Check sheet for the modelled part. Datum: model origin and axes. Units: mm. A direction names the side the tool comes from. Round coordinates to 2 decimals unless told otherwise and drop trailing zeros. Order: outer loops, then holes, each group sorted by start corner. A loop starts at its lowest first (then second) coordinate and runs counter-clockwise, first axis right, second up.
Autodesk Fusion 360 part; units mm, degrees
sketch "Sketch1" plane through (0, 0, 0) normal (0, 0, 1) x (1, 0, 0)
  line L0 (0, 0) -> (280, 0)
  line L1 (280, 0) -> (280, -8)
  line L2 (280, -8) -> (0, -8)
  line L3 (0, -8) -> (0, 0)
  dimension "d1" = 280
  dimension "d2" = 8
extrude "Extrude1" add sketch "Sketch1" along normal blind 8
sketch "Sketch2" plane through (0, 0, 0) normal (0, 0, 1) x (1, 0, 0)
  circle A0 centre (280, -4) radius 12.5
  circle A1 centre (280, -4) radius 11.3
  dimension "d5" = 25
  dimension "d6" = 22.6
extrude "Extrude2" add sketch "Sketch2" along normal blind 8
extrude "Extrude3" cut sketch "Sketch2" along normal blind 8 contours A1
extrude "Extrude4" add sketch "Sketch2" along normal blind 1.2 contours A1
fillet "Fillet1" radius 5 1 edges at (269.4647, 0.0863, 1.2)
sketch "Sketch4" plane through (0, 0, 0) normal (0, 1, 0) x (-1, 0, 0)
  line L0 (-268.1573, 8) -> (-268.1573, 0)
  line L1 (-268.1573, 0) -> (0, 0)
  line L2 (0, 0) -> (0, 8)
  line L3 (0, 8) -> (-268.1573, 8)
  circle A0 centre (-5.4, 4.0245) radius 3.45
  circle A1 centre (-21.4, 3.9983) radius 2.05
  line L4 (-21.5827, 6.0402) -> (-5.7075, 7.4608)
  line L5 (-5.6963, 0.5873) -> (-21.576, 1.9559)
  dimension "d20" = 6.9
  dimension "d21" = 5.4
  dimension "d22" = 4.1
  dimension "d23" = 16
extrude "Extrude5" cut sketch "Sketch4" against normal blind 6 contours A0 | A0 A1 L4 L5 | A1
extrude "Extrude6" cut sketch "Sketch4" against normal blind 8 contours A0
fillet "Fillet2" radius 5 1 edges at (292.5, -4, 0)
fillet "Fillet3" radius 2 1 edges at (0, -4, 8)
fillet "Fillet4" radius 2 1 edges at (0, -4, 0)
equation "d6 = 25 mm - ( 1.2 * 2 ) * 1 mm"
equation "d21 = 3.4 mm + 2 mm"
1) Set-up check for faces 1 (the face through (271.12, 2.99, 7.09)), 2 (the face through (13.76, -2.96, 6.74)), 3 (the face through (136, -3, 8)): record each of +Z, -Z, +X, -X, +Y, -Y from which the full face is reachable in a straight line by a thin tool's end or side.
2) Scan lines: line 1 (Y direction, x = 280, z = 7.5); line 2 (Z direction, x = 5.4, y = -2.5); line 3 (Y direction, x = 104, z = 1.75). Record each from-to range of solid material in increasing order.
3) Draft check along X on faces 4 (the face through (292.49, -3.51, 6.48)), 5 (the face through (280, -4, 1.2)), 6 (the face through (135, 0, 4)). Enter one of: pulls with the +X half, pulls with the -X half, needs draft (parallel to the pull), parting line crosses it, or undercut.
4) Sectioned sample at B-B on x = 135.5. Record the cut outline in (y, z).
5) Gauge pin test, flat ends, axial feed: pin 1 (4 mm diameter, centred on x = 37.5, z = 3.5, fed in from +Y); pin 2 (2.5 mm diameter, centred on x = 117.5, z = 3, fed in from -Y); pin 3 (4 mm diameter, centred on x = 277, y = -1.5, fed in from +Z). Record the tip position at first contact, or that the pin passes through.
6) Sectioned sample at A-A on x = 280. Record the cut outline in (y, z), and give its area (3 significant figures).
Values found:
1. face 1: +Z
1. face 2: +Y
1. face 3: +Z, +X, -X, +Y, -Y
2. line 1: y = -16.5 to -15.3, 7.3 to 8.5
2. line 2: z = 0 to 0.57, 7.47 to 8
2. line 3: y = -8 to 0
3. face 4: parting line crosses it
3. face 5: undercut
3. face 6: needs draft
4. outline: (-8, 0) - (0, 0) - (0, 8) - (-8, 8) - close
5. pin 1: stops at y = 0
5. pin 2: stops at y = -8
5. pin 3: stops at z = 1.2
6. outline: (-16.5, 5) arc R5 ccw to (-11.5, 0) - (3.5, 0) arc R5 ccw to (8.5, 5) - (8.5, 8) - (7.3, 8) - (7.3, 6.2) arc R5 cw to (2.3, 1.2) - (-10.3, 1.2) arc R5 cw to (-15.3, 6.2) - (-15.3, 8) - (-16.5, 8) - close
6. area: 46.3 mm2
